Autodesk Inventor part; units mm, degrees
ref_plane "YZ Plane" through (0, 0, 0) normal (1, 0, 0) x (0, 1, 0)
ref_plane "XZ Plane" through (0, 0, 0) normal (0, 1, 0) x (-1, 0, 0)
ref_plane "XY Plane" through (0, 0, 0) normal (0, 0, 1) x (1, 0, 0)
sketch "Sketch1" plane through (0, 0, 0) normal (1, 0, 0) x (0, 1, 0)
  line L0 (0, 0) -> (0, -9.398)
  line L1 (0, -9.398) -> (2.4765, -9.398)
  line L2 (9.398, -2.4765) -> (9.398, 0)
  line L3 (9.398, 0) -> (0, 0)
  line L4 (16.002, 0) -> (16.002, -2.4765)
  line L5 (22.9235, -9.398) -> (25.4, -9.398)
  line L6 (25.4, -9.398) -> (25.4, 0)
  line L7 (25.4, 0) -> (16.002, 0)
  line L8 (25.4, -16.002) -> (22.9235, -16.002)
  line L9 (16.002, -22.9235) -> (16.002, -25.4)
  line L10 (25.4, -25.4) -> (25.4, -16.002)
  line L11 (0, -16.002) -> (2.4765, -16.002)
  line L12 (9.398, -22.9235) -> (9.398, -25.4)
  line L13 (0, -25.4) -> (0, -16.002)
  line L14 (22.9235, -9.398) -> (22.9235, -4.953)
  line L15 (16.002, -2.4765) -> (20.447, -2.4765)
  line L16 (20.447, -2.4765) -> (15.0495, -7.874)
  line L17 (20.447, -2.4765) -> (28.0802, -2.4765) construction
  line L18 (22.9235, -4.953) -> (17.526, -10.3505)
  line L19 (22.9235, -16.002) -> (22.9235, -20.447)
  line L20 (22.9235, -20.447) -> (17.526, -15.0495)
  line L21 (16.002, -22.9235) -> (20.447, -22.9235)
  line L22 (20.447, -22.9235) -> (15.0495, -17.526)
  line L23 (2.4765, -16.002) -> (2.4765, -20.447)
  line L24 (2.4765, -20.447) -> (7.874, -15.0495)
  line L25 (9.398, -22.9235) -> (4.953, -22.9235)
  line L26 (4.953, -22.9235) -> (10.3505, -17.526)
  line L27 (9.398, -2.4765) -> (4.953, -2.4765)
  line L28 (4.953, -2.4765) -> (10.3505, -7.874)
  line L29 (2.4765, -9.398) -> (2.4765, -4.953)
  line L30 (2.4765, -4.953) -> (7.874, -10.3505)
  line L31 (10.3505, -7.874) -> (15.0495, -7.874)
  line L32 (17.526, -10.3505) -> (17.526, -15.0495)
  line L33 (10.3505, -17.526) -> (15.0495, -17.526)
  line L34 (7.874, -15.0495) -> (7.874, -10.3505)
  circle A0 centre (12.7, -12.7) radius 2.54
  line L35 (0, -50.8) -> (0, -41.402)
  line L36 (0, -41.402) -> (2.4765, -41.402)
  line L37 (9.398, -48.3235) -> (9.398, -50.8)
  line L38 (9.398, -50.8) -> (0, -50.8)
  line L39 (16.002, -50.8) -> (16.002, -48.3235)
  line L40 (22.9235, -41.402) -> (25.4, -41.402)
  line L41 (25.4, -41.402) -> (25.4, -50.8)
  line L42 (25.4, -50.8) -> (16.002, -50.8)
  line L43 (25.4, -34.798) -> (22.9235, -34.798)
  line L44 (16.002, -27.8765) -> (16.002, -25.4)
  line L45 (25.4, -25.4) -> (25.4, -34.798)
  line L46 (0, -34.798) -> (2.4765, -34.798)
  line L47 (9.398, -27.8765) -> (9.398, -25.4)
  line L48 (0, -25.4) -> (0, -34.798)
  line L49 (22.9235, -41.402) -> (22.9235, -45.847)
  line L50 (16.002, -48.3235) -> (20.447, -48.3235)
  line L51 (20.447, -48.3235) -> (15.0495, -42.926)
  line L52 (20.447, -48.3235) -> (28.0802, -48.3235) construction
  line L53 (22.9235, -45.847) -> (17.526, -40.4495)
  line L54 (22.9235, -34.798) -> (22.9235, -30.353)
  line L55 (22.9235, -30.353) -> (17.526, -35.7505)
  line L56 (16.002, -27.8765) -> (20.447, -27.8765)
  line L57 (20.447, -27.8765) -> (15.0495, -33.274)
  line L58 (2.4765, -34.798) -> (2.4765, -30.353)
  line L59 (2.4765, -30.353) -> (7.874, -35.7505)
  line L60 (9.398, -27.8765) -> (4.953, -27.8765)
  line L61 (4.953, -27.8765) -> (10.3505, -33.274)
  line L62 (9.398, -48.3235) -> (4.953, -48.3235)
  line L63 (4.953, -48.3235) -> (10.3505, -42.926)
  line L64 (2.4765, -41.402) -> (2.4765, -45.847)
  line L65 (2.4765, -45.847) -> (7.874, -40.4495)
  line L66 (10.3505, -42.926) -> (15.0495, -42.926)
  line L67 (17.526, -40.4495) -> (17.526, -35.7505)
  line L68 (10.3505, -33.274) -> (15.0495, -33.274)
  line L69 (7.874, -35.7505) -> (7.874, -40.4495)
  circle A1 centre (12.7, -38.1) radius 2.54
  dimension "d2" = 9.398
  dimension "d3" = 2.4765
  dimension "d7" = 2.4765
  dimension "d10" = 2.4765
  dimension "d11" = 25.4
  dimension "d13" = 2.4765
  dimension "d16" = 2.4765
  dimension "d17" = 9.398
  dimension "d23" = 2.4765
  dimension "d25" = 25.4
  dimension "d32" = 4.445
  dimension "d33" = 4.445
  dimension "d35" = 135
  dimension "d36" = 4.445
  dimension "d37" = 4.445
  dimension "d38" = 2.4765
  dimension "d40" = 4.445
  dimension "d41" = 4.445
  dimension "d42" = 4.445
  dimension "d43" = 4.445
  dimension "d44" = 5.08
extrude "Extrusion1" add sketch "Sketch1" along normal blind 127
properties part number "LatX24in1"
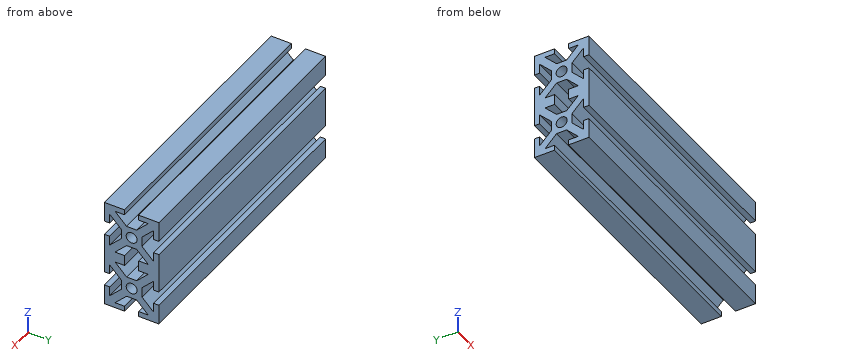
Build history of the part. All positions in model axes, mm. Round coordinates to 2 decimals unless told otherwise and drop trailing zeros. Loops run counter-clockwise (first coordinate to the right, second up) from the corner with the lowest first, then second, coordinate; pieces in that order, holes last.
Item 1: Saw through at A-A (y = 12.7). List the corners of the cut face in (x, z), then the cut area to 3 significant figures.
Item 2: Drill centre lines: line 1 along Z through (x, y) = (93, 1.5); line 2 along Z through (x, y) = (72, 12.7); line 3 along Z through (x, y) = (115, 14.75). Where is each one in solid material? Low to high.
Item 3: Pin check, flat tips, straight feed: P1, Ø2, axis at x = 90, z = -1, coming from the -Y side; P2, Ø4, axis at x = 70, z = -11.5, coming from the -Y side; P3, Ø1.4, axis at x = 54.5, z = -11.5, coming from the +Y side; P4, Ø4, axis at x = 43.5, z = -38, coming from the -Y side. Stop position of each tip, or through.
Item 4: Saw through at C-C (x = 72). State how many separate pieces and enclosed holes the cut face has, then the cut area to 3 significant figures.
Item 5: Saw through at B-B (z = -12.7). List the corners of the cut face in (x, y).
Worked answers:
1. outline: (0, -42.93) - (127, -42.93) - (127, -40.64) - (0, -40.64) - close; (0, -35.56) - (127, -35.56) - (127, -33.27) - (0, -33.27) - close; (0, -17.53) - (127, -17.53) - (127, -15.24) - (0, -15.24) - close; (0, -10.16) - (127, -10.16) - (127, -7.87) - (0, -7.87) - close
1. area: 1,160 mm2
2. line 1: z = -50.8 to -41.4, -34.8 to -16, -9.4 to 0
2. line 2: z = -42.93 to -40.64, -35.56 to -33.27, -17.53 to -15.24, -10.16 to -7.87
2. line 3: z = -42.93 to -39.6, -36.6 to -33.27, -17.53 to -14.2, -11.2 to -7.87
3. P1: stops at y = 0
3. P2: stops at y = 7.02
3. P3: stops at y = 17.53
3. P4: stops at y = 7.87
4. separate pieces: 1
4. enclosed holes: 3
4. area: 683 mm2
5. outline: (0, 7.87) - (127, 7.87) - (127, 10.16) - (0, 10.16) - close; (0, 15.24) - (127, 15.24) - (127, 17.53) - (0, 17.53) - close
